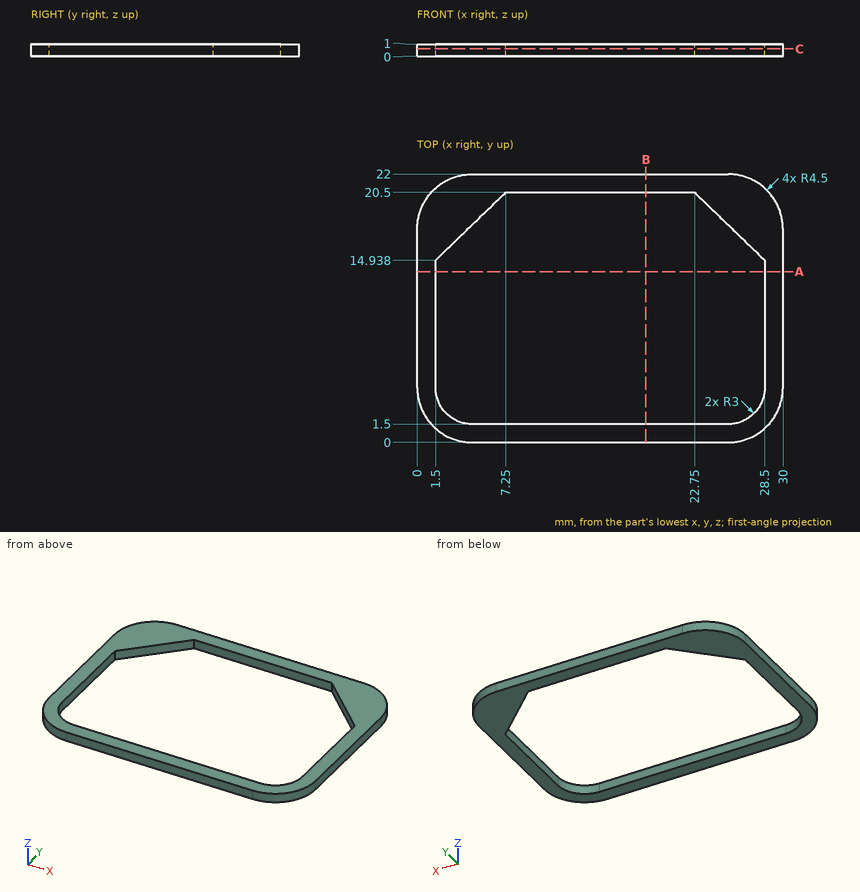
Can you work these out from the drawing? Everything is in mm from the part's minimum corner. Give positions to 0.01 mm unless a question says otherwise; leave off trailing zeros. Loops run counter-clockwise (first coordinate to the right, second up) from the corner with the lowest first, then second, coordinate; pieces in that order, holes last. Notation, with made-up numbers: M -20.5,-10.5 L 19.5,-10.5 A17 cw 19.5,4.5 Z; hole C 16,2.5 d5. An arc over 180 degrees is marked long. Put each result on its own line as item: value. Start each with the question number.
(1) I want a section at C-C on z = 0.6. Please give me the cut outline in (x, y).
(2) I need wall thicknesses on line 1 along Y through (x, z) = (17, 0.95); line 2 along X through (y, z) = (13, 0.6); line 3 along Y through (x, z) = (25.75, 0.85). Which ranges of each line are inside material? Lowest first, please. Write a range as [from, to].
(3) I want a section at B-B on x = 18.75. Please give me the cut outline in (y, z).
(4) I want a section at A-A on y = 14. Please give me the cut outline in (x, z), then the cut area to 3 significant figures.
Answer block:
1. outline: M 0,4.5 A4.5 ccw 4.5,0 L 25.5,0 A4.5 ccw 30,4.5 L 30,17.5 A4.5 ccw 25.5,22 L 4.5,22 A4.5 ccw 0,17.5 Z; hole M 1.5,4.5 A3 ccw 4.5,1.5 L 25.5,1.5 A3 ccw 28.5,4.5 L 28.5,14.94 L 22.75,20.5 L 7.25,20.5 L 1.5,14.94 Z
2. line 1: [0, 1.5], [20.5, 22]
2. line 2: [0, 1.5], [28.5, 30]
2. line 3: [0.01, 1.51], [17.6, 21.99]
3. outline: M 0,0 L 1.5,0 L 1.5,1 L 0,1 Z; M 20.5,0 L 22,0 L 22,1 L 20.5,1 Z
4. outline: M 0,0 L 1.5,0 L 1.5,1 L 0,1 Z; M 28.5,0 L 30,0 L 30,1 L 28.5,1 Z
4. area: 3.00 mm^2
